Design review of the part built by this model. Coordinates are the model's own, in mm. Give positions to 0.01 mm unless a question says otherwise; leave off trailing zeros. Write each loop counter-clockwise with the first axis right and the second up, starting at its lowest first coordinate (ties: lowest second). Pieces come first, ordered by that corner, then holes. Notation, with made-up numbers: M -33.75,18 L -11.75,18 A25 cw -11.75,54 Z; hole C -35,82.25 d8. An arc over 180 degrees is marked long. Answer in a Markdown table with one row per item.
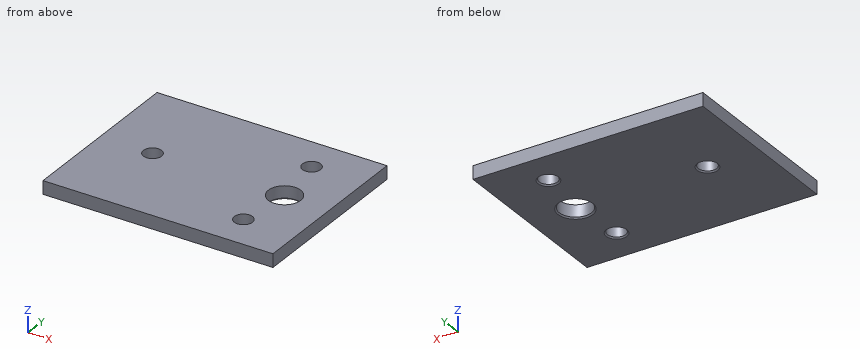
```python
from build123d import *

# Parameters (mm, degrees)
ESQUISSE2_W                        = 110
ESQUISSE2_H                        = 85
BOSS_EXTRU_1_DEPTH                 = 3.175
F_5_16_CLEARANCE_HOLE1_D           = 8.72998
F_5_16_CLEARANCE_HOLE1_CSINK_D     = 9.99998
F_5_16_CLEARANCE_HOLE1_CSINK_ANGLE = 90


with BuildPart() as part:
    # Esquisse2 → Boss.-Extru.1 (new, symmetric)
    with BuildSketch(Plane.XY):
        Rectangle(ESQUISSE2_W, ESQUISSE2_H)
    extrude(amount=BOSS_EXTRU_1_DEPTH, both=True)

    # 5/16 Clearance Hole1 (through all)
    with Locations(Plane(origin=(0, 0, -3.175), x_dir=(-1, 0, 0), z_dir=(0, 0, -1))):
        with Locations((-29.89199, 25.4), (-29.89199, -25.4), (29.89199, 0)):
            CounterSinkHole(F_5_16_CLEARANCE_HOLE1_D / 2, F_5_16_CLEARANCE_HOLE1_CSINK_D / 2, counter_sink_angle=F_5_16_CLEARANCE_HOLE1_CSINK_ANGLE)

    # Sketch4 → 9/16 Clearance Hole1 (revolve, cut)
    with BuildSketch(Plane(origin=(33.26638, 0, -3.175), x_dir=(0, 1, 0), z_dir=(1, 0, 0))):
        Polygon((0, 0), (0, 6.35), (7.73938, 6.35), (7.73938, 0.635), (8.37438, 0), align=None)
    revolve(axis=Axis((33.26638, 0, -9.525), (0, 0, 1)), mode=Mode.SUBTRACT)


solid = part.part
```
1) Add section A-A (y = 0). Write out the cut boundary in (x, z) (3 decimals), and give its area (3 significant figures).
Geometry says:
| item | result |
|---|---|
| outline | M -55,-3.175 L -34.892,-3.175 L -34.257,-2.54 L -34.257,3.175 L -55,3.175 Z; M -25.527,-2.54 L -24.892,-3.175 L 24.892,-3.175 L 25.527,-2.54 L 25.527,3.175 L -25.527,3.175 Z; M 41.006,-2.54 L 41.641,-3.175 L 55,-3.175 L 55,3.175 L 41.006,3.175 Z |
| area | 544 mm^2 |
2) To check wall thickness, follow probe 1 along X at (y, z) = (0, -1.4); probe 2 along Y at (x, z) = (26.5, -1.5); probe 3 along Y at (x, z) = (27.5, -0.75). State the ranges of each line that lie inside material, in increasing order. Write a range as [from, to].
Geometry says:
| item | result |
|---|---|
| probe 1 | [-55, -34.26], [-25.53, 25.53], [41.01, 55] |
| probe 2 | [-42.5, -28.15], [-22.65, -3.76], [3.76, 22.65], [28.15, 42.5] |
| probe 3 | [-42.5, -29.05], [-21.75, -5.16], [5.16, 21.75], [29.05, 42.5] |
3) Add section C-C (z = 0). Write out the cut boundary in (x, y).
Geometry says:
| item | result |
|---|---|
| outline | M -55,-42.5 L 55,-42.5 L 55,42.5 L -55,42.5 Z; hole C -29.89,0 d8.73; hole C 29.89,-25.4 d8.73; hole C 33.27,0 d15.48; hole C 29.89,25.4 d8.73 |
4) Add section B-B (y = 25.4). Write out the cut boundary in (x, z) (3 decimals).
Geometry says:
| item | result |
|---|---|
| outline | M -55,-3.175 L 24.892,-3.175 L 25.527,-2.54 L 25.527,3.175 L -55,3.175 Z; M 34.257,-2.54 L 34.892,-3.175 L 55,-3.175 L 55,3.175 L 34.257,3.175 Z |
